The listing builds one solid part. Answer for the finished solid, in the listing's coordinates (mm). A direction names the side the tool comes from. Give positions to 0.01 mm unless a question says otherwise; leave off trailing zeros. Order: outer loops, then holes, each group sorted by start corner. A loop starts at its lowest first (then second) coordinate and runs counter-clockwise, first axis right, second up. Notation, with made-up numbers: M 80.5,21.25 L 126.5,21.25 A20 ccw 126.5,35.25 Z; hole C 21,74.25 d6. An arc over 180 degrees is marked long. Answer as a JSON object with one key per item and string values. Group by question number.
```python
from build123d import *

# Parameters (mm, degrees)
F0_W     = 220
F0_H     = 40
F1_DEPTH = 2
F2_W     = 10.18609
F2_H     = 40
F3_DEPTH = 7
F5_DEPTH = 2
F7_DEPTH = 40.001


with BuildPart() as f1:
    # F0 (on Top) → F1 (new body)
    with BuildSketch(Plane.XY):
        with Locations((49.58334, 5.469682)):
            Rectangle(F0_W, F0_H)
    extrude(amount=F1_DEPTH)

    # F2 (on face) → F3 (join)
    with BuildSketch(Plane(origin=(0, 0, 0), x_dir=(1, 0, 0), z_dir=(0, 0, -1))):
        with Locations((-55.323615, -5.469682)):
            Rectangle(F2_W, F2_H)
    extrude(amount=F3_DEPTH)

    # F4 (on face) → F5 (join)
    with BuildSketch(Plane.XY.offset(2)):
        Polygon((159.58334, 25.469682), (-60.41666, 25.469682), (-60.41666, -14.530318), (159.58334, -14.530318), (159.58334, -12.530318), (-57.984237, -12.530318), (-57.984237, 23.469682), (159.58334, 23.469682), align=None)
    extrude(amount=F5_DEPTH)

    # F6 (on face) → F7 (cut, through all)
    with BuildSketch(Plane(origin=(0, 25.469682, 0), x_dir=(-1, 0, 0), z_dir=(0, 1, 0))):
        Polygon((50.23057, -6.4), (50.23057, -7), (60.41666, -7), align=None)
    extrude(amount=-F7_DEPTH, mode=Mode.SUBTRACT)


solid = f1.part
```
Item 1: Section C-C (z = -3.5) is taken. Determine the outline of the cut face in (x, y).
Item 2: Determine the mould class of faces 1 (the flat face through (42, 25.47, 2)), 2 (the flat face through (-60.417, 6, -2)), 3 (the flat face through (49, 6, 2)), 4 (the flat face through (41, -14.53, 2)) for opening direction Y: released by +Y, released by -Y, zero draft, split by the parting line, or undercut.
Item 3: Flat-ended cylindrical pins translate along their axes: P1, Ø2, axis at x = 84.5, y = 7.5, coming from the -Z side; P2, Ø6, axis at x = 50, y = 4.5, coming from the +Z side; P3, Ø5, axis at y = 18.5, z = -4, coming from the +X side. Find the tip coordinate at first contact, or state that the pin passes through.
Item 4: Consider probe 1 along Y at (x, z) = (-26.5, 3); probe 2 along Z at (x, y) = (43, 7.5); probe 3 along X at (y, z) = (3.5, 3.75). Determine where each line is inside the solid, lowest interval first. Write a range as from..to.
Item 5: Section B-B (x = 137.5) is taken. Determine the outline of the cut face in (y, z), and give its area (3 significant figures).
Item 6: A tool of negligible diameter and unlimited length cuts with its end or side. For faces 5 (the flat face through (53, 6, 0)), 6 (the flat face through (49, 25, 4)), from which of +Z, -Z, +X, -X, +Y, -Y can it reach the whole face along a straight path? Write none if from no direction.
Item 7: Section A-A (y = -10.5) is taken. Determine the outline of the cut face in (x, z), and give its area (3 significant figures).
Values found:
{
 "1": {"outline": "M -60.42,-14.53 L -50.23,-14.53 L -50.23,25.47 L -60.42,25.47 Z"},
 "2": {"face 1": "released by +Y", "face 2": "zero draft", "face 3": "undercut", "face 4": "released by -Y"},
 "3": {"P1": "stops at z = 0", "P2": "stops at z = 2", "P3": "stops at x = -50.23"},
 "4": {"probe 1": "y = -14.53..-12.53, 23.47..25.47", "probe 2": "z = 0..2", "probe 3": "x = -60.42..-57.98"},
 "5": {"outline": "M -14.53,0 L 25.47,0 L 25.47,4 L 23.47,4 L 23.47,2 L -12.53,2 L -12.53,4 L -14.53,4 Z", "area": "88.0 mm^2"},
 "6": {"face 5": "-Z, +X, +Y, -Y", "face 6": "+Z, +X, -X, +Y, -Y"},
 "7": {"outline": "M -60.42,-7 L -50.23,-6.4 L -50.23,0 L 159.58,0 L 159.58,2 L -57.98,2 L -57.98,4 L -60.42,4 Z", "area": "513 mm^2"}
}
